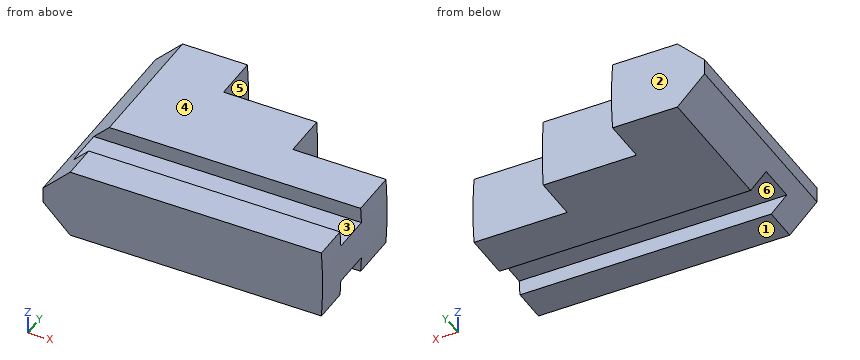
```python
from build123d import *

# Parameters (mm, degrees)
BOSS_EXTRUDE1_DEPTH = 9
SKETCH3_W           = 4
SKETCH3_H           = 10
CUT_EXTRUDE2_DEPTH  = 91.748278221
CUT_EXTRUDE3_START  = 11.6
CUT_EXTRUDE3_DEPTH  = 11.6
CUT_EXTRUDE7_DEPTH  = 11.6
CUT_EXTRUDE8_START  = -11.6
CUT_EXTRUDE8_DEPTH  = 31.3
CHAMFER1_SIZE       = 7


with BuildPart() as part:
    # Sketch1 → Boss-Extrude1 (new, symmetric)
    with BuildSketch(Plane.XY):
        Polygon((0, 0), (0, 54.5), (24, 54.5), (24, 42.9), (48, 42.9), (48, 31.3), (72, 31.3), (72, 0), align=None)
    extrude(amount=BOSS_EXTRUDE1_DEPTH, both=True)

    # Sketch3 → Cut-Extrude2 (cut, through all)
    with BuildSketch(Plane.ZY):
        with Locations((-7, 14)):
            Rectangle(SKETCH3_W, SKETCH3_H)
        with Locations((7, 14)):
            Rectangle(SKETCH3_W, SKETCH3_H)
    extrude(amount=-CUT_EXTRUDE2_DEPTH, mode=Mode.SUBTRACT)

    # Sketch4 → Cut-Extrude3 (cut)
    with BuildSketch(Plane(origin=(0, 42.9, 0), x_dir=(1, 0, 0), z_dir=(0, 1, 0)).offset(CUT_EXTRUDE3_START)):
        with BuildLine():
            Line((49.710414787, -9), (47.710414787, -9))
            ThreePointArc((47.710414787, -9), (48, 0), (47.710414787, 9))
            Line((47.710414787, 9), (49.710414787, 9))
            Line((49.710414787, 9), (49.710414787, -9))
        make_face()
        with BuildLine():
            Line((23.710414787, 9), (25.710414787, 9))
            Line((25.710414787, 9), (25.710414787, -9))
            Line((25.710414787, -9), (23.710414787, -9))
            ThreePointArc((23.710414787, -9), (24, 0), (23.710414787, 9))
        make_face()
        with BuildLine():
            Line((73.710414787, -9), (71.710414787, -9))
            ThreePointArc((71.710414787, -9), (72, 0), (71.710414787, 9))
            Line((71.710414787, 9), (73.710414787, 9))
            Line((73.710414787, 9), (73.710414787, -9))
        make_face()
    extrude(amount=-CUT_EXTRUDE3_DEPTH, mode=Mode.SUBTRACT)

    # Sketch4<3> → Cut-Extrude7 (cut)
    with BuildSketch(Plane(origin=(0, 42.9, 0), x_dir=(1, 0, 0), z_dir=(0, 1, 0))):
        with BuildLine():
            Line((49.710414787, -9), (47.710414787, -9))
            ThreePointArc((47.710414787, -9), (48, 0), (47.710414787, 9))
            Line((47.710414787, 9), (49.710414787, 9))
            Line((49.710414787, 9), (49.710414787, -9))
        make_face()
    extrude(amount=-CUT_EXTRUDE7_DEPTH, mode=Mode.SUBTRACT)

    # Sketch4<4> → Cut-Extrude8 (cut)
    with BuildSketch(Plane(origin=(0, 42.9, 0), x_dir=(1, 0, 0), z_dir=(0, 1, 0)).offset(CUT_EXTRUDE8_START)):
        with BuildLine():
            Line((73.710414787, -9), (71.710414787, -9))
            ThreePointArc((71.710414787, -9), (72, 0), (71.710414787, 9))
            Line((71.710414787, 9), (73.710414787, 9))
            Line((73.710414787, 9), (73.710414787, -9))
        make_face()
    extrude(amount=-CUT_EXTRUDE8_DEPTH, mode=Mode.SUBTRACT)

    # Chamfer1
    chamfer1_edges = [part.edges().sort_by_distance(p)[0] for p in [
        (0, 36.75, -9),
        (0, 36.75, 9),
    ]]
    chamfer(chamfer1_edges, length=CHAMFER1_SIZE)


solid = part.part
```
The model under review builds one solid part; all positions refer to its coordinate system, in mm. Face numbers are marked on the shaded views. A direction names the side the tool comes from. Give positions to 0.01 mm unless a question says otherwise; leave off trailing zeros. Write each loop counter-clockwise with the first axis right and the second up, starting at its lowest first coordinate (ties: lowest second). Pieces come first, ordered by that corner, then holes.
(1) Consider section B-B, the plane y = 34. Give the boundary of the cut face in (x, z).
(2) Consider section A-A, the plane z = 8.25. Give the boundary of the cut face in (x, y).
(3) Tool access review of the marked faces 4, 5 and 6: name each direction out of +Z, -Z, +X, -X, +Y, -Y from which nothing blocks a thin tool from reaching the whole face with its end or side.
(4) Consider section C-C, the plane x = 57.5. Give the boundary of the cut face in (y, z).
(5) To check wall thickness, follow L1, parallel to Y at x = 9.5, z = 7.5; L2, parallel to Y at x = 66.5, z = -5.5; L3, parallel to Z at x = 46, y = 14.5. State the ranges of each line that lie inside material, in increasing order.
(6) The part is to be moulded in two halves that separate along Y. For the marked faces 1, 2 and 3, say which applies: released by +Y, released by -Y, zero draft, split by the parting line, or undercut.
(7) Consider section D-D, the plane z = -3. Give the boundary of the cut face in (x, y), and give its area (3 significant figures).
(8) For P1, Ø10, axis at x = 60, z = 4.5, coming from the +Y side; P2, Ø2, axis at x = 33.5, z = 7, coming from the +Y side; P3, Ø1.5, axis at x = 31.5, y = 15.5, coming from the +Z side, all flat-tipped, find the tip position at first contact; note any pin that passes through.
Returned:
1. outline: (0, -2) - (7, -9) - (47.71, -9) arc R140 ccw to (47.71, 9) - (7, 9) - (0, 2) - close
2. outline: (6.25, 0) - (71.76, 0) - (71.76, 9) - (6.25, 9) - close; (6.25, 19) - (71.76, 19) - (71.76, 31.3) - (47.76, 31.3) - (47.76, 42.9) - (23.76, 42.9) - (23.76, 54.5) - (6.25, 54.5) - close
3. face 4: +Z, +X, -X, +Y, -Y
3. face 5: +X, +Y
3. face 6: -Z, +X, -X
4. outline: (0, -9) - (9, -9) - (9, -5) - (19, -5) - (19, -9) - (31.3, -9) - (31.3, 9) - (19, 9) - (19, 5) - (9, 5) - (9, 9) - (0, 9) - close
5. L1: y = 0 to 9, 19 to 54.5
5. L2: y = 0 to 9, 19 to 31.3
5. L3: z = -5 to 5
6. face 1: zero draft
6. face 2: released by +Y
6. face 3: undercut
7. outline: (1, 0) - (71.97, 0) - (71.97, 31.3) - (47.97, 31.3) - (47.97, 42.9) - (23.97, 42.9) - (23.97, 54.5) - (1, 54.5) - close
7. area: 3,030 mm2
8. P1: stops at y = 31.3
8. P2: stops at y = 42.9
8. P3: stops at z = 5
